Autodesk Inventor part; units mm, degrees
ref_plane "YZ Plane" through (0, 0, 0) normal (1, 0, 0) x (0, 1, 0)
ref_plane "XZ Plane" through (0, 0, 0) normal (0, 1, 0) x (-1, 0, 0)
ref_plane "XY Plane" through (0, 0, 0) normal (0, 0, 1) x (1, 0, 0)
sketch "Náčrt1" plane through (0, 0, 0) normal (0, 1, 0) x (-1, 0, 0)
  line L0 (0, 0) -> (110, 0)
  line L1 (110, 0) -> (110, -20)
  line L2 (110, -20) -> (0, -20)
  line L3 (0, -20) -> (0, 0)
  line L4 (55, -20) -> (55, 0) construction
  line L5 (110, -10) -> (0, -10) construction
  circle A0 centre (105, -10) radius 1.6
  circle A1 centre (85, -10) radius 1.6
  line L6 (105, -10) -> (105, -4.8731) construction
  line L7 (85, -10) -> (85, -4.8731) construction
  line L8 (105, -7.7373) -> (103.8686, -8.8686)
  line L9 (105, -7.7373) -> (106.1314, -8.8686)
  line L10 (85, -7.7373) -> (83.8686, -8.8686)
  line L11 (85, -7.7373) -> (86.1314, -8.8686)
  dimension "d0" = 20
  dimension "d1" = 110
  dimension "d4" = 3.2
  dimension "d6" = 25
  dimension "d7" = 5
  dimension "d49" = 90
  dimension "d50" = 90
extrude "Vysunutí1" add sketch "Náčrt1" along normal blind 16
sketch "Náčrt2" plane through (0, 16, 0) normal (0, 1, 0) x (1, 0, 0)
  line L0 (0, 20) -> (-110, 20)
  line L1 (-110, 20) -> (-110, 0)
  line L2 (-110, 0) -> (0, 0)
  line L3 (0, 0) -> (0, 20)
  arc A0 (-83.8686, 8.8686) -> (-86.1314, 8.8686) centre (-85, 10) ccw
  arc A1 (-103.8686, 8.8686) -> (-106.1314, 8.8686) centre (-105, 10) ccw
  line L4 (-80, 0) -> (-80, 20)
  line L5 (-30, 0) -> (-30, 20)
  arc A2 (-103.8686, 8.8686) -> (-106.1314, 8.8686) centre (-105, 10) ccw construction
  arc A3 (-83.8686, 8.8686) -> (-86.1314, 8.8686) centre (-85, 10) ccw
  line L6 (-85, 7.7373) -> (-86.1314, 8.8686)
  line L7 (-83.8686, 8.8686) -> (-85, 7.7373)
  line L8 (-105, 7.7373) -> (-106.1314, 8.8686)
  line L9 (-103.8686, 8.8686) -> (-105, 7.7373)
  point P0 (0, 10)
  point P1 (-30, 10)
  point P2 (-85, 7.7373)
  point P3 (-105, 7.7373)
  dimension "d10" = 30
  dimension "d11" = 30
extrude "Vysunutí2" cut sketch "Náčrt2" against normal blind 11 contours L4 L2 L1 L0 | L7 L6 A0 | L9 L8 A1
sketch "Náčrt4" plane through (0, 0, 0) normal (0, -1, 0) x (1, 0, 0)
  line L0 (0, -20) -> (-110, -20)
  line L1 (0, 0) -> (0, -20)
  line L2 (-110, 0) -> (0, 0)
  line L3 (-110, -20) -> (-110, 0)
  arc A0 (-86.1314, -8.8686) -> (-83.8686, -8.8686) centre (-85, -10) ccw
  arc A1 (-106.1314, -8.8686) -> (-103.8686, -8.8686) centre (-105, -10) ccw
  arc A2 (-110, -20) -> (-110, -20) centre (-105, -10) ccw
  line L4 (-105, -6.8246) -> (-102.25, -8.4123)
  line L5 (-102.25, -8.4123) -> (-102.25, -11.5877)
  line L6 (-102.25, -11.5877) -> (-105, -13.1754)
  line L7 (-105, -13.1754) -> (-107.75, -11.5877)
  line L8 (-107.75, -11.5877) -> (-107.75, -8.4123)
  line L9 (-107.75, -8.4123) -> (-105, -6.8246)
  arc A3 (-110, -20) -> (-110, -20) centre (-85, -10) ccw
  line L10 (-84.9134, -6.8258) -> (-82.2077, -8.4879)
  line L11 (-82.2077, -8.4879) -> (-82.2943, -11.6621)
  line L12 (-82.2943, -11.6621) -> (-85.0866, -13.1742)
  line L13 (-85.0866, -13.1742) -> (-87.7923, -11.5121)
  line L14 (-87.7923, -11.5121) -> (-87.7057, -8.3379)
  line L15 (-87.7057, -8.3379) -> (-84.9134, -6.8258)
  line L16 (-85, -7.7373) -> (-86.1314, -8.8686)
  line L17 (-83.8686, -8.8686) -> (-85, -7.7373)
  line L18 (-105, -7.7373) -> (-106.1314, -8.8686)
  line L19 (-103.8686, -8.8686) -> (-105, -7.7373)
  point P0 (-102.25, -10)
  point P1 (-107.75, -10)
  dimension "d17" = 5.5
extrude "Vysunutí4" cut sketch "Náčrt4" against normal blind 2.5 contours L16 L17 A0 | L18 L19 A1 | L4 L5 L6 L7 L8 L9 | L10 L11 L12 L13 L14 L15
sketch "Náčrt6" plane through (-110, 0, 0) normal (0, 0, 1) x (1, 0, 0)
  line L0 (0, 0) -> (0, 5)
  line L1 (0, 0) -> (110, 0)
  line L2 (110, 0) -> (110, 16)
  line L3 (30, 16) -> (110, 16)
  line L4 (110, 16) -> (0, 16)
  line L5 (80, 16) -> (80, 0)
  line L6 (30, 16) -> (30, 5)
  line L7 (30, 5) -> (0, 5)
  dimension "d24" = 30
extrude "Vysunutí5" cut sketch "Náčrt6" against normal blind 10 contours L5 L3 L2 L1
sketch "Náčrt7" plane through (-110, 0, -10) normal (0, 0, 1) x (1, 0, 0)
  line L0 (80, 16) -> (110, 16)
  line L1 (80, 0) -> (80, 16)
  line L2 (110, 0) -> (80, 0)
  line L3 (110, 16) -> (110, 0)
  line L4 (110, 0) -> (110, 16) construction
  line L5 (110, 8) -> (80, 8) construction
  circle A0 centre (85, 8) radius 1.6
  circle A1 centre (105, 8) radius 1.6
  line L6 (85, 8) -> (85, 12.494) construction
  line L7 (105, 8) -> (105, 11.0554) construction
  line L8 (85, 10.2627) -> (83.8686, 9.1314)
  line L9 (85, 10.2627) -> (86.1314, 9.1314)
  line L10 (105, 10.2627) -> (103.8686, 9.1314)
  line L11 (105, 10.2627) -> (106.1314, 9.1314)
  dimension "d30" = 3.2
  dimension "d31" = 25
  dimension "d32" = 5
  dimension "d38" = 90
  dimension "d39" = 90
extrude "Vysunutí6" cut sketch "Náčrt7" against normal through all contours A0 | A1
sketch "Náčrt8" plane through (0, 0, -20) normal (0, 0, -1) x (-1, 0, 0)
  circle A0 centre (5, 8) radius 1.6
  circle A1 centre (25, 8) radius 1.6
  line L0 (0, 16) -> (80, 16)
  line L1 (0, 0) -> (0, 16)
  line L2 (0, 0) -> (110, 0)
  line L3 (110, 0) -> (110, 5)
  line L4 (25, 4.8246) -> (22.25, 6.4123)
  line L5 (22.25, 6.4123) -> (22.25, 9.5877)
  line L6 (22.25, 9.5877) -> (25, 11.1754)
  line L7 (25, 11.1754) -> (27.75, 9.5877)
  line L8 (27.75, 9.5877) -> (27.75, 6.4123)
  line L9 (27.75, 6.4123) -> (25, 4.8246)
  line L10 (5, 4.8246) -> (2.25, 6.4123)
  line L11 (2.25, 6.4123) -> (2.25, 9.5877)
  line L12 (2.25, 9.5877) -> (5, 11.1754)
  line L13 (5, 11.1754) -> (7.75, 9.5877)
  line L14 (7.75, 9.5877) -> (7.75, 6.4123)
  line L15 (7.75, 6.4123) -> (5, 4.8246)
  line L16 (80, 5) -> (80, 16)
  line L17 (110, 5) -> (80, 5)
  dimension "d35" = 5.5
extrude "Vysunutí7" cut sketch "Náčrt8" against normal blind 2.5 contours A0 | A1 | L4 L5 L6 L7 L8 L9 | L10 L11 L12 L13 L14 L15
sketch "Náčrt10" plane through (-110, 5, 0) normal (0, 0, 1) x (1, 0, 0)
  line L0 (80, -5) -> (80, 11)
  line L1 (30, 11) -> (80, 11)
  line L2 (0, -5) -> (0, 0)
  line L3 (0, -5) -> (80, -5)
  circle A0 centre (105, 3) radius 1.6
  circle A1 centre (85, 3) radius 1.6
  line L4 (80, 11) -> (110, 11)
  line L5 (80, -5) -> (80, 11)
  line L6 (110, -5) -> (80, -5)
  line L7 (110, 11) -> (110, -5)
  line L8 (55, 22.3819) -> (55, -13.3022) construction
  line L9 (110, -5) -> (110, 11) construction
  line L10 (110, 3) -> (22.1304, 3) construction
  line L11 (35, 3) -> (75, 3) construction
  line L12 (35, 1.5) -> (75, 1.5)
  line L13 (75, 4.5) -> (35, 4.5)
  arc A2 (35, 4.5) -> (35, 1.5) centre (35, 3) ccw
  arc A3 (75, 1.5) -> (75, 4.5) centre (75, 3) ccw
  line L14 (110, -5) -> (0, -5)
  line L15 (30, 11) -> (30, 0)
  line L16 (30, 0) -> (0, 0)
  point P0 (55, 3)
  point P1 (55, -5)
  dimension "d43" = 3
  dimension "d44" = 40
extrude "Vysunutí8" cut sketch "Náčrt10" against normal up to surface (20 mm away) contours A2 L13 A3 L12
chamfer "Zkosení3" distance 0.5 angle 45 18 edges at (-70, 0, 0) (-55, 0, -20) (-55, 16, 0) (-110, 2.5, 0) (-110, 2.5, -20) (-110, 0, -10) (0, 0, -15) (0, 8, -20) (0, 16, -15) (-40, 16, -20) (-55, 6.5, 0) (-76.5, 8, 0) (-55, 9.5, 0) (-33.5, 8, 0) (-55, 6.5, -20) (-33.5, 8, -20) (-55, 9.5, -20) (-76.5, 8, -20)
properties part number "middle_hole"
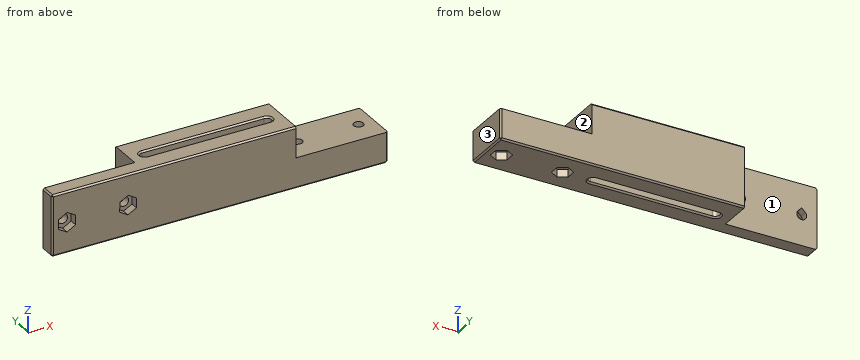
The model under review builds one solid part; all positions refer to its coordinate system, in mm. Face numbers are marked on the shaded views. A direction names the side the tool comes from. Round coordinates to 2 decimals unless told otherwise and drop trailing zeros. Write each loop counter-clockwise with the first axis right and the second up, starting at its lowest first coordinate (ties: lowest second). Pieces come first, ordered by that corner, then holes. Notation, with made-up numbers: M 67,12.5 L 93,12.5 A28 cw 93,41.5 Z; hole C 81,47 d5. An arc over 180 degrees is marked long. Use a Markdown table: item, result. Add a question column.
Q1. Insertion check: pin 1 (1 mm diameter, centred on x = -18.5, y = 7.5, fed in from +Z); pin 2 (4 mm diameter, centred on y = 7.5, z = -12.5, fed in from -X); pin 3 (3 mm diameter, centred on y = 8, z = -4, fed in from +X). Each pin has a flat end and moves straight along its axis. Give the tip position at first contact, or say it passes through.
Q2. Machinability: for the marked faces 1, 2 and 3, which of the approach directions +Z, -Z, +X, -X, +Y, -Y give a long, thin tool a straight path to every point of the face, cutting with its end or side? Answer none if there is none.
Q3. We need section C-C, the plane z = -3.75. State the section outline as (x, y) points, plus the area to 3 significant figures.
Q4. To check wall thickness, follow line 1 (X direction, y = 8, z = -15); line 2 (Y direction, x = -61, z = -9.5); line 3 (Y direction, x = -25, z = -13.25). State the ranges of each line that lie inside material, in increasing order.
Q5. We need section D-D, the plane x = -9. State the section outline as (y, z) points.
Q6. We need section B-B, the plane y = 12.5. State the section outline as (x, z) points.
Q7. We need section A-A, the plane x = -70. State the section outline as (y, z) points, plus the area to 3 significant figures.
Findings below:
| question | item | result |
|---|---|---|
| 1 | pin 1 | stops at z = -10 |
| 1 | pin 2 | stops at x = -80 |
| 1 | pin 3 | stops at x = -30 |
| 2 | face 1 | +Z, -Z, -X, +Y |
| 2 | face 2 | +Z, +X, +Y, -Y |
| 2 | face 3 | +Z, -Z, +X, +Y, -Y |
| 3 | outline | M -110,0.5 L -109.5,0 L -30,0 L -30,16 L -80,16 L -80,5 L -110,5 Z; hole M -75,6.5 L -35,6.5 A1.5 ccw -35,9.5 L -75,9.5 A1.5 ccw Z |
| 3 | area | 823 mm² |
| 4 | line 1 | x = -80 to -76.5, -33.5 to -26.6, -23.4 to -6.6, -3.4 to 0 |
| 4 | line 2 | y = 0 to 6.5, 9.5 to 16 |
| 4 | line 3 | y = 0 to 6.4, 9.6 to 16 |
| 5 | outline | M 0,-19.5 L 0.5,-20 L 15.5,-20 L 16,-19.5 L 16,-10 L 0,-10 Z |
| 6 | outline | M -80,-20 L -0.5,-20 L 0,-19.5 L 0,-10 L -30,-10 L -30,0 L -80,0 Z |
| 7 | outline | M 0,-19.5 L 0.5,-20 L 6,-20 L 6.5,-19.5 L 6.5,-0.5 L 6,0 L 0.5,0 L 0,-0.5 Z; M 9.5,-19.5 L 10,-20 L 15.5,-20 L 16,-19.5 L 16,-0.5 L 15.5,0 L 10,0 L 9.5,-0.5 Z |
| 7 | area | 259 mm² |
